from build123d import *

# Parameters (mm, degrees)
F0_W     = 85
F0_H     = 85
F0_R     = 2.75
F0_R_2   = 37.85
F1_DEPTH = 20
F2_W     = 20
F2_H     = 10
F3_DEPTH = 40
F4_R     = 3.25
F5_DEPTH = 10.001
F6_SIZE  = 3


with BuildPart() as f1:
    # F0 (on Top) → F1 (new body)
    with BuildSketch(Plane.XY):
        Rectangle(F0_W, F0_H)
        with Locations((-37, -37)):
            Circle(F0_R, mode=Mode.SUBTRACT)
        with Locations((37, -37)):
            Circle(F0_R, mode=Mode.SUBTRACT)
        with Locations((-37, 37)):
            Circle(F0_R, mode=Mode.SUBTRACT)
        Circle(F0_R_2, mode=Mode.SUBTRACT)
        with Locations((37, 37)):
            Circle(F0_R, mode=Mode.SUBTRACT)
    extrude(amount=F1_DEPTH)

    # F2 (on Top) → F3 (join)
    with BuildSketch(Plane.XY):
        with Locations((-52.5, -37.5)):
            Rectangle(F2_W, F2_H)
        with Locations((52.5, -37.5)):
            Rectangle(F2_W, F2_H)
    extrude(amount=F3_DEPTH)

    # F4 (on face) → F5 (cut, through all)
    with BuildSketch(Plane(origin=(0, -32.5, 0), x_dir=(-1, 0, 0), z_dir=(0, 1, 0))):
        with Locations((-52.5, 20)):
            Circle(F4_R)
        with Locations((52.5, 20)):
            Circle(F4_R)
    extrude(amount=-F5_DEPTH, mode=Mode.SUBTRACT)

    # F6
    f6_edges = [f1.edges().sort_by_distance(p)[0] for p in [
        (-42.5, 42.5, 10),
        (42.5, 42.5, 10),
    ]]
    chamfer(f6_edges, length=F6_SIZE)


solid = f1.part
For this review, take the finished solid that the model builds, in its own axes (mm). A direction names the side the tool comes from. Round coordinates to 2 decimals unless told otherwise and drop trailing zeros. Order: outer loops, then holes, each group sorted by start corner. A loop starts at its lowest first (then second) coordinate and runs counter-clockwise, first axis right, second up. Notation, with made-up numbers: M 87.5,-22 L 108.5,-22 A11 ccw 108.5,-3 Z; hole C -30,-12.75 d8. An arc over 180 degrees is marked long. Write each question's results on one line, items separated by ' | '. Start each with the question number.
1. Add section B-B (y = 0). State the section outline as (x, z) points.
2. Clearance check with flat-ended pins moving along their axes: pin 1 Ø22 at (x, z) = (56.5, 25.5) entering from +Y; pin 2 Ø4.5 at (x, y) = (-37, 37) entering from -Z; pin 3 Ø10 at (x, y) = (38.5, -28) entering from +Z; pin 4 Ø10 at (y, z) = (-12.5, 14.5) entering from +X. State where each tip first meets the part, or that it passes through.
3. Tool access review of faces 1 (the face through (-42.5, -38, 30)), 2 (the face through (-53, -37, 40)): name each direction out of +Z, -Z, +X, -X, +Y, -Y from which nothing blocks a thin tool from reaching the whole face with its end or side.
4. Add section D-D (x = -36). State the section outline as (y, z) points.
5. Draft analysis for pull direction X (two halves, no side actions). For faces 3 (the face through (48, -32.5, 20)), 4 (the face through (42.5, 3, 10)), 5 (the face through (36.1, 11.37, 9.86)), 6 (the face through (-39.027, -35.141, 9.86)), state which applies: pulls with the +X half, pulls with the -X half, needs draft (parallel to the pull), parting line crosses it, or undercut.
6. To check wall thickness, follow L1, parallel to Z at x = 52.5, y = -37.25; L2, parallel to Y at x = 35, z = 18.5; L3, parallel to X at y = -36.5, z = 36. State the ranges of each line that lie inside material, in increasing order. Write a range as [from, to].
7. Add section C-C (z = 35). State the section outline as (x, y) points, then the cut area to 3 significant figures.
8. Add section A-A (z = 2.5). State the section outline as (x, y) points.
Output values:
1) outline: M -42.5,0 L -37.85,0 L -37.85,20 L -42.5,20 Z; M 37.85,0 L 42.5,0 L 42.5,20 L 37.85,20 Z
2) pin 1: y = -32.5 | pin 2: through | pin 3: z = 20 | pin 4: x = 42.5
3) face 1: +Z, +Y, -Y | face 2: +Z, +X, -X, +Y, -Y
4) outline: M -42.5,0 L -39.56,0 L -39.56,20 L -42.5,20 Z; M -34.44,0 L -11.69,0 L -11.69,20 L -34.44,20 Z; M 11.69,0 L 34.44,0 L 34.44,20 L 11.69,20 Z; M 39.56,0 L 42.5,0 L 42.5,20 L 39.56,20 Z
5) face 3: needs draft | face 4: pulls with the +X half | face 5: undercut | face 6: undercut
6) L1: [0, 16.75], [23.25, 40] | L2: [-42.5, -38.89], [-35.11, -14.41], [14.41, 35.11], [38.89, 42.5] | L3: [-62.5, -42.5], [42.5, 62.5]
7) outline: M -62.5,-42.5 L -42.5,-42.5 L -42.5,-32.5 L -62.5,-32.5 Z; M 42.5,-42.5 L 62.5,-42.5 L 62.5,-32.5 L 42.5,-32.5 Z | area: 400 mm^2
8) outline: M -62.5,-42.5 L 62.5,-42.5 L 62.5,-32.5 L 42.5,-32.5 L 42.5,39.5 L 39.5,42.5 L -39.5,42.5 L -42.5,39.5 L -42.5,-32.5 L -62.5,-32.5 Z; hole C -37,-37 d5.5; hole C -37,37 d5.5; hole C 0,0 d75.7; hole C 37,-37 d5.5; hole C 37,37 d5.5
